from build123d import *

# Parameters (mm, degrees)
SKETCH2_W           = 300
SKETCH2_H           = 300
BOSS_EXTRUDE1_DEPTH = 10
SKETCH3_W           = 30
SKETCH3_H           = 60
BOSS_EXTRUDE2_DEPTH = 130
FILLET1_R           = 30
SKETCH4_R           = 30
BOSS_EXTRUDE4_DEPTH = 60
BOSS_EXTRUDE5_START = 60
SKETCH5_R           = 30
BOSS_EXTRUDE5_DEPTH = 60
BOSS_EXTRUDE6_START = -40
BOSS_EXTRUDE6_DEPTH = 40
BOSS_EXTRUDE7_DEPTH = 40
SKETCH8_R           = 15.05
CUT_EXTRUDE1_DEPTH  = 40
SKETCH9_R           = 15.05
CUT_EXTRUDE2_DEPTH  = 40
FILLET2_R           = 15


with BuildPart() as part:
    # Sketch2 → Boss-Extrude1 (new body)
    with BuildSketch(Plane(origin=(0, 0, 0), x_dir=(1, 0, 0), z_dir=(0, 1, 0))):
        Rectangle(SKETCH2_W, SKETCH2_H)
    extrude(amount=BOSS_EXTRUDE1_DEPTH)

    # Sketch3 → Boss-Extrude2 (add)
    with BuildSketch(Plane(origin=(0, 10, 0), x_dir=(1, 0, 0), z_dir=(0, 1, 0))):
        with Locations((-125, 0)):
            Rectangle(SKETCH3_W, SKETCH3_H)
        with Locations((125, 0)):
            Rectangle(SKETCH3_W, SKETCH3_H)
    extrude(amount=BOSS_EXTRUDE2_DEPTH)

    # Fillet1
    fillet1_edges = [part.edges().sort_by_distance(p)[0] for p in [
        (125, 140, -30),
        (125, 140, 30),
        (-125, 140, 30),
        (-125, 140, -30),
    ]]
    fillet(fillet1_edges, radius=FILLET1_R - 0.0001)  # a hair under: the kernel refuses the full size

    # Sketch4 → Boss-Extrude4 (add)
    with BuildSketch(Plane.ZY.offset(140)):
        with Locations((0, 110)):
            Circle(SKETCH4_R)
    extrude(amount=BOSS_EXTRUDE4_DEPTH)

    # Sketch5 → Boss-Extrude5 (add)
    with BuildSketch(Plane(origin=(140, 0, 0), x_dir=(0, 0, -1), z_dir=(1, 0, 0)).offset(BOSS_EXTRUDE5_START)):
        with Locations((0, 110)):
            Circle(SKETCH5_R)
    extrude(amount=-BOSS_EXTRUDE5_DEPTH)

    # Sketch6 → Boss-Extrude6 (add)
    with BuildSketch(Plane.ZY.offset(200).offset(BOSS_EXTRUDE6_START)):
        with BuildLine():
            Line((-21.895741175, 89.492037683), (-58.637033052, 79.647238196))
            Line((-58.637033052, 79.647238196), (-68.637033052, 116.967746272))
            Line((-68.637033052, 116.967746272), (-23.070072037, 129.177376677))
            ThreePointArc((-23.070072037, 129.177376677), (-29.986874166, 109.112656899), (-21.895741175, 89.492037683))
        make_face()
        with BuildLine():
            Line((21.768001871, 89.356499945), (57.587704831, 76.319194267))
            Line((57.587704831, 76.319194267), (70.443457025, 111.640083129))
            Line((70.443457025, 111.640083129), (23.412322022, 128.758016354))
            ThreePointArc((23.412322022, 128.758016354), (29.973910166, 108.749116558), (21.768001871, 89.356499945))
        make_face()
    extrude(amount=BOSS_EXTRUDE6_DEPTH)

    # Sketch7 → Boss-Extrude7 (add)
    with BuildSketch(Plane(origin=(200, 0, 0), x_dir=(0, 0, -1), z_dir=(1, 0, 0))):
        with BuildLine():
            Line((-21.768001871, 89.356499945), (-57.587704831, 76.319194267))
            Line((-57.587704831, 76.319194267), (-70.443457025, 111.640083129))
            Line((-70.443457025, 111.640083129), (-23.412322022, 128.758016354))
            ThreePointArc((-23.412322022, 128.758016354), (-29.973910166, 108.749116558), (-21.768001871, 89.356499945))
        make_face()
        with BuildLine():
            Line((23.070072037, 129.177376677), (68.637033052, 116.967746272))
            Line((68.637033052, 116.967746272), (58.637033052, 79.647238196))
            Line((58.637033052, 79.647238196), (21.895741175, 89.492037683))
            ThreePointArc((21.895741175, 89.492037683), (29.986874166, 109.112656899), (23.070072037, 129.177376677))
        make_face()
    extrude(amount=-BOSS_EXTRUDE7_DEPTH)

    # Sketch8 → Cut-Extrude1 (cut)
    with BuildSketch(Plane(origin=(0, -9.323904974, -34.797287089), x_dir=(-1, 0, 0), z_dir=(0, -0.2588190451025219, -0.965925826289068))):
        with Locations(Location((-180, 111.428221794, 0), (0, 0, 90))):
            Circle(SKETCH8_R)
    cut_extrude1 = extrude(amount=-CUT_EXTRUDE1_DEPTH, mode=Mode.SUBTRACT)

    # Mirror1: Cut-Extrude1 across plane
    add(cut_extrude1.mirror(Plane(origin=(0, 0, 0), x_dir=(0, 0, 1), z_dir=(1, 0, 0))), mode=Mode.SUBTRACT)

    # Sketch9 → Cut-Extrude2 (cut)
    with BuildSketch(Plane(origin=(0, -9.58068177, 26.322706827), x_dir=(1, 0, 0), z_dir=(0, -0.3420201433256628, 0.9396926207859106))):
        with Locations(Location((180, 110.206591153, 0), (0, 0, 270))):
            Circle(SKETCH9_R)
    cut_extrude2 = extrude(amount=-CUT_EXTRUDE2_DEPTH, mode=Mode.SUBTRACT)

    # Mirror2: Cut-Extrude2 across plane
    add(cut_extrude2.mirror(Plane(origin=(0, 0, 0), x_dir=(0, 0, 1), z_dir=(1, 0, 0))), mode=Mode.SUBTRACT)

    # Fillet2
    fillet2_edges = [part.edges().sort_by_distance(p)[0] for p in [
        (160, 120.199049742, 46.927889523),
        (160, 82.837847106, 39.677853351),
        (200, 120.199049742, 46.927889523),
        (200, 82.837847106, 39.677853351),
        (160, 84.569637939, -40.266387113),
        (160, 123.072561474, -45.853552544),
        (200, 123.072561474, -45.853552544),
        (200, 84.569637939, -40.266387113),
        (-160, 123.072561474, -45.853552544),
        (-160, 84.569637939, -40.266387113),
        (-200, 84.569637939, -40.266387113),
        (-200, 123.072561474, -45.853552544),
        (-160, 82.837847106, 39.677853351),
        (-160, 120.199049742, 46.927889523),
        (-200, 120.199049742, 46.927889523),
        (-200, 82.837847106, 39.677853351),
    ]]
    fillet(fillet2_edges, radius=FILLET2_R)


solid = part.part
The model under review builds one solid part; all positions refer to its coordinate system, in mm. A direction names the side the tool comes from. Round coordinates to 2 decimals unless told otherwise and drop trailing zeros. Write each loop counter-clockwise with the first axis right and the second up, starting at its lowest first coordinate (ties: lowest second). Pieces come first, ordered by that corner, then holes. Notation, with made-up numbers: (-23, -14) -> (6, -14) arc R20 cw to (6, -6) -> close; hole circle Ø7 at (38, 59.25). An arc over 180 degrees is marked (long way). Answer as a JSON object with one key per item and string values.
1. We need section D-D on x = 39. State the section outline as (y, z) points.
Results found:
{"outline": "(0, -150) -> (10, -150) -> (10, 150) -> (0, 150) -> close"}
2. To check wall thickness, follow line 1 along X through (y, z) = (83, 4.5); line 2 along Y through (x, z) = (-108, -73); line 3 along X through (y, z) = (106, 57). State the ranges of each line that lie inside material, in increasing order.
Results found:
{"line 1": "x = -200 to -110, 110 to 200", "line 2": "y = 0 to 10", "line 3": "x = -199.11 to -192.14, -167.86 to -160.89, 160.89 to 167.86, 192.14 to 199.11"}
3. Clearance check with flat-ended pins moving along their axes: pin 1 (24 mm diameter, centred on x = -118.5, y = 38.5, fed in from +Z); pin 2 (24 mm diameter, centred on x = -130.5, y = 77, fed in from -Z); pin 3 (3 mm diameter, centred on y = 94.5, z = 36.5, fed in from +X). State where each tip first meets the part, or that it passes through.
Results found:
{"pin 1": "stops at z = 30", "pin 2": "stops at z = -30", "pin 3": "stops at x = 199.55"}
4. The part is to be moulded in two halves that separate along Y. For faces 4 (the face through (-140, 48, 0)), 5 (the face through (-179.93, 82.93, 39.43)), 6 (the face through (-195.72, 116.08, 45.06)), 7 (the face through (125, 59, 30)), say which applies: pulls with the +Y half, pulls with the -Y half, needs draft (parallel to the pull), parting line crosses it, or undercut.
Results found:
{"face 4": "undercut", "face 5": "pulls with the -Y half", "face 6": "pulls with the +Y half", "face 7": "needs draft"}
5. We need section C-C on z = 105.5. State the section outline as (x, y) points, and give its area (3 significant figures).
Results found:
{"outline": "(-150, 0) -> (150, 0) -> (150, 10) -> (-150, 10) -> close", "area": "3,000 mm^2"}
6. We need section B-B on z = 43.5. State how many separate pieces and enclosed holes the cut face has, and give its area (3 significant figures).
Results found:
{"separate pieces": "3", "enclosed holes": "2", "area": "4,270 mm^2"}
7. Machinability: for faces 1 (the face through (125, 59, -30)), 2 (the face through (-195.49, 86.77, 41.39)), 3 (the face through (-125, 59, 30)), which of the approach directions +Z, -Z, +X, -X, +Y, -Y give a long, thin tool a straight path to every point of the face, cutting with its end or side? Answer none if there is none.
Results found:
{"face 1": "-Z, +Y", "face 2": "-X, -Y", "face 3": "+Z, +Y"}
8. We need section A-A on y = 35. State the section outline as (x, z) points.
Results found:
{"outline": "(-140, -30) -> (-110, -30) -> (-110, 30) -> (-140, 30) -> close; (110, -30) -> (140, -30) -> (140, 30) -> (110, 30) -> close"}
